```python
from build123d import *

# Parameters (mm, degrees)
F0_R     = 40
F1_DEPTH = 0.4
F2_W     = 44.7093093119
F2_H     = 48.3685829416
F3_DEPTH = 25


with BuildPart() as f1:
    # F0 (on Top) → F1 (new body)
    with BuildSketch(Plane.XY):
        Circle(F0_R)
    extrude(amount=F1_DEPTH)

    # F2 (on face) → F3 (cut)
    with BuildSketch(Plane.XY.offset(0.4)):
        Rectangle(F2_W, F2_H)
        with BuildLine():
            Line((-27.354654656, -22.2321893938), (-27.354654656, 22.2321893938))
            ThreePointArc((-27.354654656, 22.2321893938), (-35.2497854829, 0), (-27.354654656, -22.2321893938))
        make_face()
        with BuildLine():
            ThreePointArc((19.7692819277, 29.1842914708), (0, 35.2497854829), (-19.7692819277, 29.1842914708))
            Line((-19.7692819277, 29.1842914708), (19.7692819277, 29.1842914708))
        make_face()
        with BuildLine():
            ThreePointArc((35.2497854829, 0), (33.2174132434, 11.7962211748), (27.354654656, 22.2321893938))
            Line((27.354654656, 22.2321893938), (27.354654656, -22.2321893938))
            ThreePointArc((27.354654656, -22.2321893938), (33.2174132434, -11.7962211748), (35.2497854829, 0))
        make_face()
        with BuildLine():
            Line((19.7692819277, -29.1842914708), (-19.7692819277, -29.1842914708))
            ThreePointArc((-19.7692819277, -29.1842914708), (0, -35.2497854829), (19.7692819277, -29.1842914708))
        make_face()
    extrude(amount=-F3_DEPTH, mode=Mode.SUBTRACT)


solid = f1.part
```
Build history of the part. All positions in model axes, mm. Coordinates: 2 decimals unless noted, no trailing zeros. Order: outer loops, then holes, each group sorted by start corner. A loop starts at its lowest first (then second) coordinate and runs counter-clockwise, first axis right, second up. Notation, with made-up numbers: M 34.5,52 L 66.5,52 A22 cw 66.5,62 Z; hole C -0.75,79 d1. An arc over 180 degrees is marked long. One line per question, with ' | ' between items. Start each with the question number.
1. Cut at A-A (z = 0.3). Write the cut outline in (x, y).
2. Cut at B-B (x = 0). Write the cut outline in (y, z).
3. Flat gauge pin, fed straight in: P1, Ø6, axis at x = 11, y = -30, coming from the -Z side. Where does the tip first touch, or does it go through?
4. Cut at D-D (y = -12.5). Write the cut outline in (x, z), plus the area to 3 significant figures.
5. Mould opens along X. For faces 1 (the face through (26, 1, 0)), 2 (the face through (-0.29, -35.25, 0.2)), 3 (the face through (-8.67, -39.05, 0.2)) say: +X half, -X half, draft (parallel to the pull), parting line (faces both ways), or undercut.
6. Wall check: line 1 along Y through (x, z) = (-12.5, 0.1); line 2 along Y through (x, z) = (-5, 0.35); line 3 along X through (y, z) = (10.5, 0.35). Give the ranges that are in metal, low to high. Write a range as [from, to].
7. Cut at C-C (y = 30.5). Write the cut outline in (x, z), plus the area to 3 significant figures.
The answers:
1) outline: C 0,0 d80; hole M -27.35,-22.23 L -27.35,22.23 A35.25 ccw Z; hole M -22.35,-24.18 L 22.35,-24.18 L 22.35,24.18 L -22.35,24.18 Z; hole M -19.77,-29.18 A35.25 ccw 19.77,-29.18 Z; hole M -19.77,29.18 L 19.77,29.18 A35.25 ccw Z; hole M 27.35,-22.23 A35.25 ccw 27.35,22.23 Z
2) outline: M -40,0 L -35.25,0 L -35.25,0.4 L -40,0.4 Z; M -29.18,0 L -24.18,0 L -24.18,0.4 L -29.18,0.4 Z; M 24.18,0 L 29.18,0 L 29.18,0.4 L 24.18,0.4 Z; M 35.25,0 L 40,0 L 40,0.4 L 35.25,0.4 Z
3) P1: stops at z = 0
4) outline: M -38,0 L -32.96,0 L -32.96,0.4 L -38,0.4 Z; M -27.35,0 L -22.35,0 L -22.35,0.4 L -27.35,0.4 Z; M 22.35,0 L 27.35,0 L 27.35,0.4 L 22.35,0.4 Z; M 32.96,0 L 38,0 L 38,0.4 L 32.96,0.4 Z | area: 8.03 mm2
5) face 1: draft | face 2: undercut | face 3: parting line
6) line 1: y = [-38, -32.96], [-29.18, -24.18], [24.18, 29.18], [32.96, 38] | line 2: y = [-39.69, -34.89], [-29.18, -24.18], [24.18, 29.18], [34.89, 39.69] | line 3: x = [-38.6, -33.65], [-27.35, -22.35], [22.35, 27.35], [33.65, 38.6]
7) outline: M -25.88,0 L -17.67,0 L -17.67,0.4 L -25.88,0.4 Z; M 17.67,0 L 25.88,0 L 25.88,0.4 L 17.67,0.4 Z | area: 6.57 mm2
